Source: three-view drawing plus pictorial views. Frame: mm from the lowest corner of the part. A direction names the side the tool comes from. Give positions to 0.01 mm unless a question says otherwise; leave off trailing zeros. Loops run counter-clockwise (first coordinate to the right, second up) from the corner with the lowest first, then second, coordinate; pieces in that order, holes last.
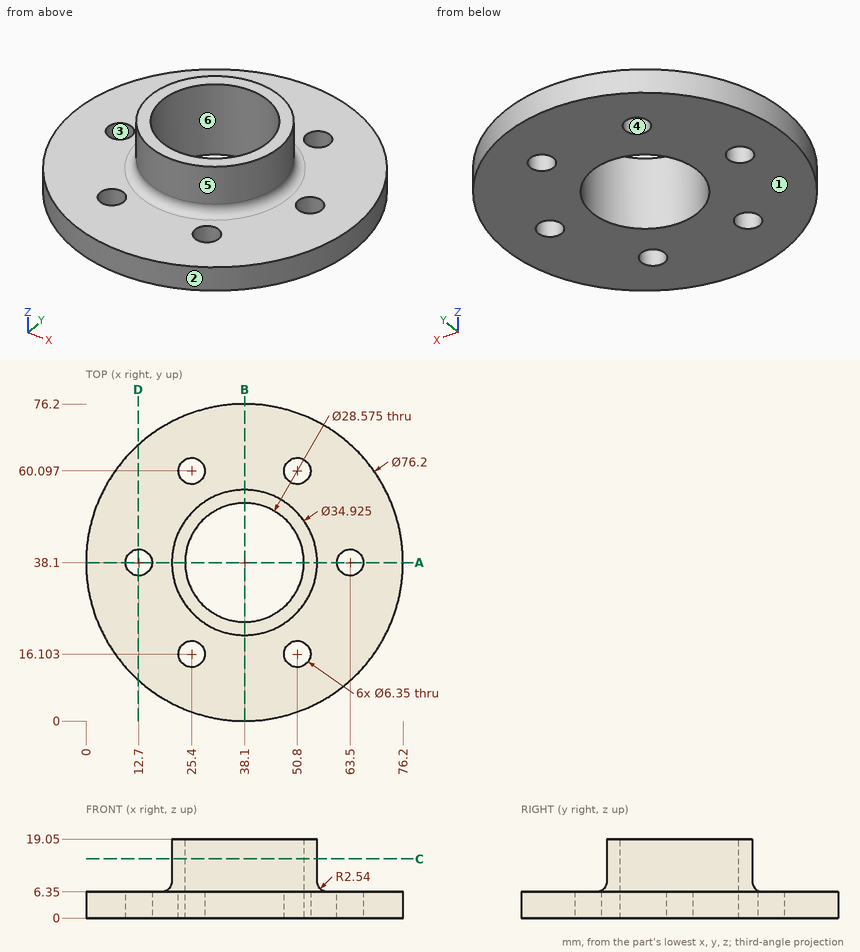
1) Cut plane D-D (x = 12.5). Return loops of the section in (y, z), and give its area (3 significant figures).
Checks:
outline: (9.88, 0) - (34.93, 0) - (34.93, 6.35) - (9.88, 6.35) - close; (41.27, 0) - (66.32, 0) - (66.32, 6.35) - (41.27, 6.35) - close
area: 318 mm2
2) Ray query, probe 1 along X at (y, z) = (39, 4); probe 2 along Y at (x, z) = (50.8, 2) (1 decimal); probe 3 along Z at (x, y) = (60.5, 23.5). Return the intervals inside material, ascending.
Checks:
probe 1: x = 0.01 to 9.66, 15.74 to 23.84, 52.36 to 60.46, 66.54 to 76.19
probe 2: y = 2.2 to 12.9, 19.3 to 31.6, 44.6 to 56.9, 63.3 to 74
probe 3: z = 0 to 6.35
3) Cut plane C-C (z = 14.25). Return loops of the section in (x, y) (1 decimal), and give its area (3 significant figures).
Checks:
outline: circle Ø34.9 at (38.1, 38.1); hole circle Ø28.6 at (38.1, 38.1)
area: 317 mm2
4) Contact query for flat-ended pins moving along their axis: P1, Ø10, axis at x = 63.5, y = 38.1, coming from the +Z side; P2, Ø5.5, axis at x = 12.7, y = 38.1, coming from the +Z side; P3, Ø8, axis at x = 12, z = 8, coming from the -Y side; P4, Ø6, axis at y = 54.5, z = 4, coming from the +X side. Output: stop coordinate, or through.
Checks:
P1: stops at z = 6.35
P2: passes through
P3: stops at y = 7.32
P4: stops at x = 73.77
5) Cut plane B-B (x = 38.1). Return loops of the section in (y, z), and give its area (3 significant figures).
Checks:
outline: (0, 0) - (23.81, 0) - (23.81, 19.05) - (20.64, 19.05) - (20.64, 8.89) arc R2.54 cw to (18.1, 6.35) - (0, 6.35) - close; (52.39, 0) - (76.2, 0) - (76.2, 6.35) - (58.1, 6.35) arc R2.54 cw to (55.56, 8.89) - (55.56, 19.05) - (52.39, 19.05) - close
area: 386 mm2
6) Cut plane A-A (y = 38.1). State how many separate pieces and enclosed holes the cut face has, and give its area (3 significant figures).
Checks:
separate pieces: 4
enclosed holes: 0
area: 305 mm2
7) Pull-direction query (X, two-part tool) for the marked faces 1, 2, 3 and 4; classes: released by +X, released by -X, zero draft, split by the parting line, or undercut.
Checks:
face 1: zero draft
face 2: split by the parting line
face 3: undercut
face 4: undercut
8) Reachability of the marked faces 5 and 6 from +Z, -Z, +X, -X, +Y, -Y: full face, straight path, thin tool, end or side. Return the list, or none.
Checks:
face 5: +Z
face 6: +Z, -Z
